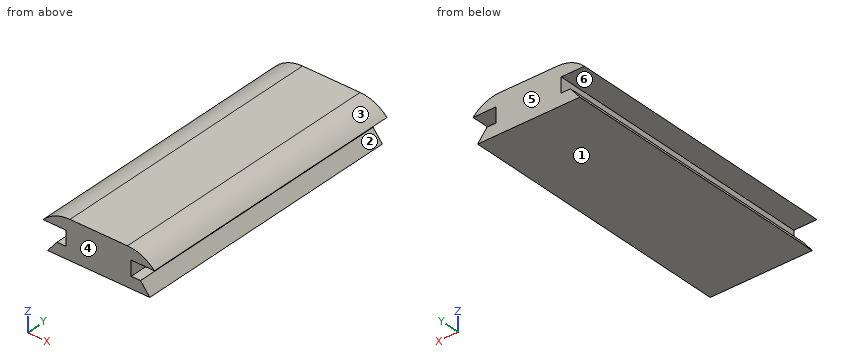
```python
from build123d import *

# Parameters (mm, degrees)
F0_W        = 35
F0_H        = 8
F1_DEPTH    = 150
F2_T1_DEPTH = 197.5947518654


# Not quite as in the source:
# - a fillet or chamfer that OpenCascade refuses, or shapes differently, is made with other operations: its cross-section is extruded or revolved along the edge and cut away or added


with BuildPart() as f1:
    # F0 (on Front) → F1 (new body)
    with BuildSketch(Plane.XZ):
        with Locations((17.5, 4)):
            Rectangle(F0_W, F0_H)
        Polygon((35, 0), (0, 0), (-5, 0), (-10, -6.2449979984), (45, -6.2449979984), (40, 0), align=None)
        Polygon((-12.5, 8), (0, 8), (35, 8), (47.5, 8), (42.5, 14.2449979984), (-7.5, 14.2449979984), align=None)
    extrude(amount=F1_DEPTH)

    # F2: fillet of radius 20 on 2 edges, made by hand

    # F2_s2 → F2_t1 (cut)
    with BuildSketch(Plane.XZ.offset(-23.7973759327)):
        with BuildLine():
            ThreePointArc((2.0189503731, 14.2449979984), (-5.8835796005, 12.6175323912), (-12.5, 8))
            Line((-12.5, 8), (-7.5, 14.2449979984))
            Line((-7.5, 14.2449979984), (2.0189503731, 14.2449979984))
        make_face()
        with BuildLine():
            ThreePointArc((47.5, 8), (40.8835796005, 12.6175323912), (32.9810496269, 14.2449979984))
            Line((32.9810496269, 14.2449979984), (42.5, 14.2449979984))
            Line((42.5, 14.2449979984), (47.5, 8))
        make_face()
    extrude(amount=F2_T1_DEPTH, mode=Mode.SUBTRACT)


solid = f1.part
```
Design review of the part built by this model. Coordinates are the model's own, in mm. Face numbers are marked on the shaded views. A direction names the side the tool comes from. Coordinates: 2 decimals unless noted, no trailing zeros. Loops run counter-clockwise (first coordinate to the right, second up) from the corner with the lowest first, then second, coordinate; pieces in that order, holes last. Notation, with made-up numbers: (19, 27.5) -> (30, 27.5) arc R15 cw to (30, 46.5) -> close; hole circle Ø11 at (40.5, 81). An arc over 180 degrees is marked (long way). Answer as a JSON object with one key per item and string values.
Q1. Clearance check with flat-ended pins moving along their axes: pin 1 Ø4 at (y, z) = (-91, 5.5) entering from +X; pin 2 Ø5.5 at (x, y) = (-2.5, -49.5) entering from +Z; pin 3 Ø9 at (y, z) = (-103, 3) entering from -X. State where each tip first meets the part, or that it passes through.
Answer block:
{"pin 1": "stops at x = 35", "pin 2": "stops at z = 14.17", "pin 3": "stops at x = -6.2"}
Q2. Take a section at C-C on z = 3. Give the boundary of the cut face in (x, y), plus the area to 3 significant figures.
Answer block:
{"outline": "(0, -150) -> (35, -150) -> (35, 0) -> (0, 0) -> close", "area": "5,250 mm^2"}
Q3. To check wall thickness, follow L1, parallel to X at y = -58.5, z = 0.25; L2, parallel to Z at x = -1.5, y = -131.5 (3 decimals); L3, parallel to Z at x = 41, y = -126 (3 decimals). State the ranges of each line that lie inside material, in increasing order.
Answer block:
{"L1": "x = 0 to 35", "L2": "z = -6.245 to 0, 8 to 13.933", "L3": "z = -6.245 to -1.249, 8 to 12.567"}
Q4. Take a section at A-A on x = 37.5. Give the boundary of the cut face in (y, z) (3 decimals).
Answer block:
{"outline": "(-150, -6.245) -> (0, -6.245) -> (0, 0) -> (-150, 0) -> close; (-150, 8) -> (0, 8) -> (0, 13.728) -> (-150, 13.728) -> close"}
Q5. Take a section at B-B on y = -28.5. Give the boundary of the cut face in (x, z) (3 decimals), plus the area to 3 significant figures.
Answer block:
{"outline": "(-12.5, 8) -> (0, 8) -> (0, 0) -> (-5, 0) -> (-10, -6.245) -> (45, -6.245) -> (40, 0) -> (35, 0) -> (35, 8) -> (47.5, 8) arc R20 ccw to (32.981, 14.245) -> (2.019, 14.245) arc R20 ccw to start", "area": "911 mm^2"}
Q6. The part is to be moulded in two halves that separate along Z. For the marked faces 1, 2, 3 and 4, say which applies: +Z half, -Z half, draft (parallel to the pull), parting line (faces both ways), or undercut.
Answer block:
{"face 1": "-Z half", "face 2": "undercut", "face 3": "+Z half", "face 4": "draft"}
Q7. Tool access review of the marked faces 5 and 6: name each direction out of +Z, -Z, +X, -X, +Y, -Y from which nothing blocks a thin tool from reaching the whole face with its end or side.
Answer block:
{"face 5": "+Z, -Z, +X, -X, +Y", "face 6": "-X, +Y, -Y"}
Q8. Take a section at D-D on x = -2. Give the boundary of the cut face in (y, z) (3 decimals).
Answer block:
{"outline": "(-150, -6.245) -> (0, -6.245) -> (0, 0) -> (-150, 0) -> close; (-150, 8) -> (0, 8) -> (0, 13.837) -> (-150, 13.837) -> close"}
